Check sheet for the drawn part. Datum: minimum x, y, z corner. Units: mm. Give positions to 0.01 mm unless a question says otherwise; leave off trailing zeros. Loops run counter-clockwise (first coordinate to the right, second up) from the corner with the lowest first, then second, coordinate; pieces in that order, holes last.
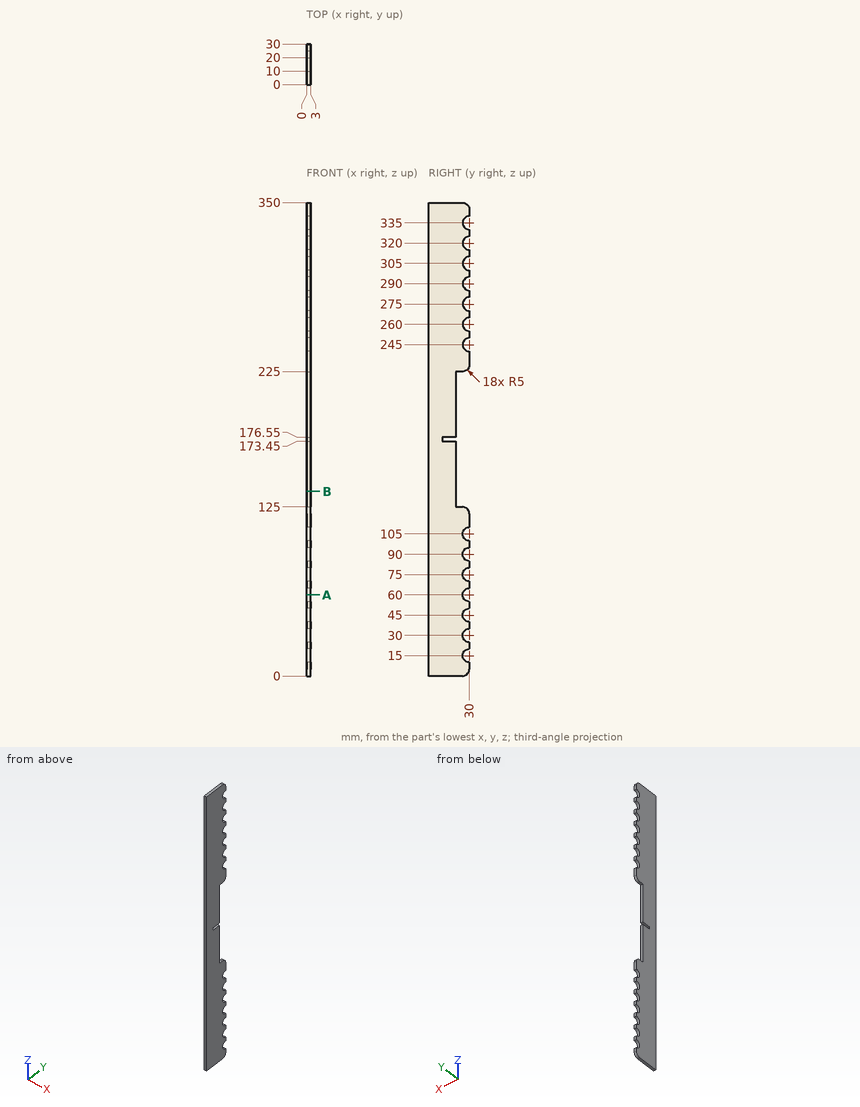
1) Depth check by flat-ended pin: P1, Ø1.5, axis at y = 17, z = 109.5, coming from the -X side; P2, Ø1.5, axis at x = 2, z = 175, coming from the +Y side. Enter the tip coordinate at first touch or a pass-through.
2) Scan lines: line 1 along Z through (x, y) = (2.75, 10.5); line 2 along Z through (x, y) = (0.1, 23.75); line 3 along Y through (x, z) = (0.7, 175). Record each from-to range of solid material in increasing order.
3) Sectioned sample at A-A on z = 60. Enter the section's corners in (x, y), plus the area to 3 significant figures.
4) Sectioned sample at B-B on z = 136.5. Enter the section's corners in (x, y), plus the area to 3 significant figures.
Determined:
1. P1: stops at x = 0
1. P2: stops at y = 10
2. line 1: z = 0 to 173.45, 176.55 to 350
2. line 2: z = 0 to 125, 225 to 350
2. line 3: y = 0 to 10
3. outline: (0, 0) - (3, 0) - (3, 25) - (0, 25) - close
3. area: 75.0 mm2
4. outline: (0, 0) - (3, 0) - (3, 20) - (0, 20) - close
4. area: 60.0 mm2
